The drawing under review shows one solid part. Ordinate dimensions are in mm from its lowest x, y, z. Give positions to 0.01 mm unless a question says otherwise; leave off trailing zeros. Write each loop counter-clockwise with the first axis right and the second up, starting at its lowest first coordinate (ties: lowest second). Pieces come first, ordered by that corner, then holes. Notation, with made-up numbers: (59, 52.5) -> (63, 52.5) arc R25 cw to (63, 75.5) -> close; hole circle Ø2 at (43, 35). An arc over 180 degrees is marked (long way). Write item = value, one per line.
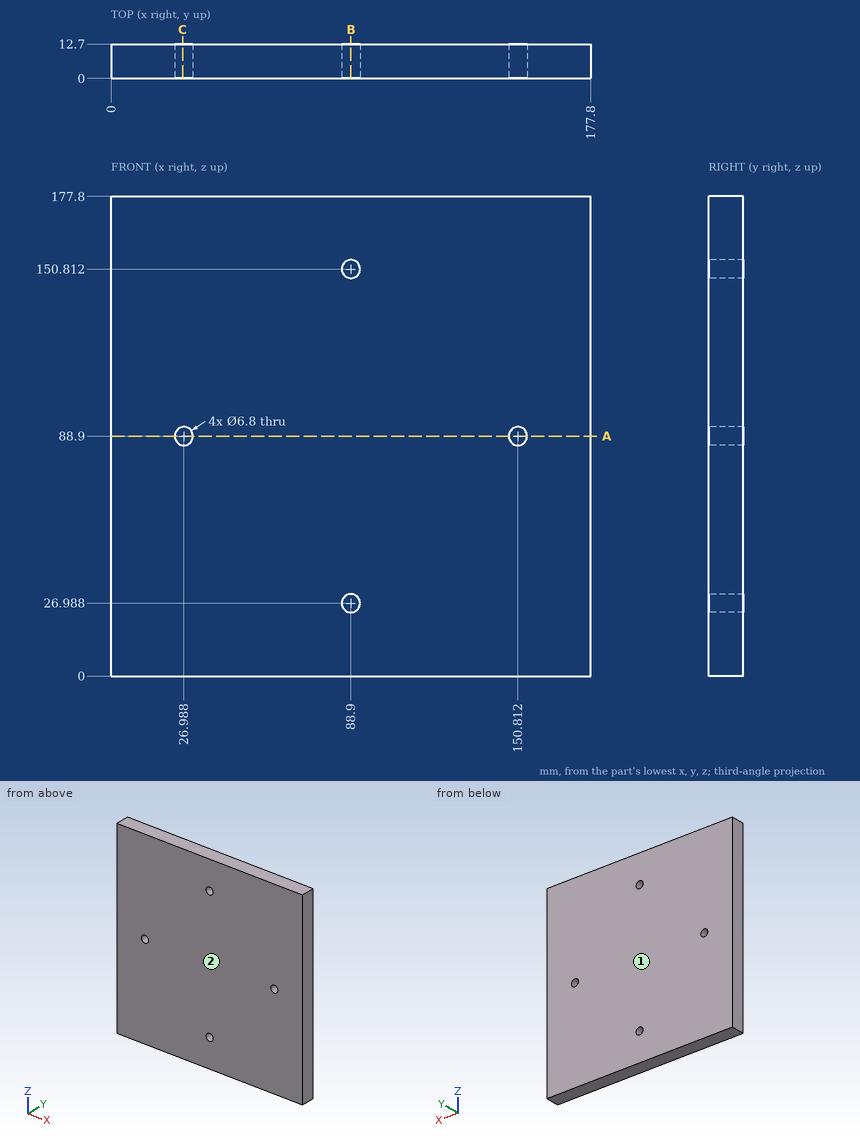
(1) To check wall thickness, follow probe 1 along Z at (x, y) = (88.9, 4.75); probe 2 along Z at (x, y) = (27, 3.75). State the ranges of each line that lie inside material, in increasing order.
Answers below:
probe_1 = 0 to 23.59, 30.39 to 147.41, 154.21 to 177.8
probe_2 = 0 to 85.5, 92.3 to 177.8
(2) For pin 1 (11 mm diameter, centred on x = 88.9, z = 26.99, fed in from -Y), flat-tipped, find the tip position at first contact; note if it passes through.
Answers below:
pin_1 = 0
(3) Take a section at C-C (x = 26.5). Write out the cut boundary in (y, z) (1 decimal).
Answers below:
outline = (0, 0) -> (12.7, 0) -> (12.7, 85.5) -> (0, 85.5) -> close; (0, 92.3) -> (12.7, 92.3) -> (12.7, 177.8) -> (0, 177.8) -> close
(4) Take a section at A-A (z = 88.9). Write out the cut boundary in (x, y).
Answers below:
outline = (0, 0) -> (23.59, 0) -> (23.59, 12.7) -> (0, 12.7) -> close; (30.39, 0) -> (147.41, 0) -> (147.41, 12.7) -> (30.39, 12.7) -> close; (154.21, 0) -> (177.8, 0) -> (177.8, 12.7) -> (154.21, 12.7) -> close
(5) The part is to be moulded in two halves that separate along Y. For the marked faces 1 and 2, say which applies: released by +Y, released by -Y, zero draft, split by the parting line, or undercut.
Answers below:
face_1 = released by +Y
face_2 = released by -Y
(6) Take a section at B-B (x = 88.9). Write out the cut boundary in (y, z).
Answers below:
outline = (0, 0) -> (12.7, 0) -> (12.7, 23.59) -> (0, 23.59) -> close; (0, 30.39) -> (12.7, 30.39) -> (12.7, 147.41) -> (0, 147.41) -> close; (0, 154.21) -> (12.7, 154.21) -> (12.7, 177.8) -> (0, 177.8) -> close
